Design review of the part built by this model. Coordinates are the model's own, in mm. A direction names the side the tool comes from. Coordinates: 2 decimals unless noted, no trailing zeros. Order: outer loops, then holes, each group sorted by start corner. A loop starts at its lowest first (then second) coordinate and runs counter-clockwise, first axis right, second up. Notation, with made-up numbers: (-15.75, 72.25) -> (23.25, 72.25) arc R17 cw to (23.25, 91.25) -> close; hole circle Ø11 at (-36, 1). An arc over 180 degrees is marked (long way). Use a Markdown table: item, result. Add a question column.
Q1. The part is to be moulded in two halves that separate along X. For faces 4 (the face through (4, 2, 42.9)), 5 (the face through (21.43, 1.68, 23.85)), 6 (the face through (12, 0, 2)), say which applies: pulls with the +X half, pulls with the -X half, needs draft (parallel to the pull), parting line crosses it, or undercut.
Q2. Add section D-D (x = 0.5). Count the separate pieces of the cut face and the enclosed holes in it, then the cut area to 3 significant figures.
Q3. Machinability: for faces 1 (the face through (9.61, 7.53, 23.77)), 2 (the face through (14, -2, 3.5)), 3 (the face through (24, 0, 34.2)), which of the approach directions +Z, -Z, +X, -X, +Y, -Y give a long, thin tool a straight path to every point of the face, cutting with its end or side? Answer none if there is none.
Q4. Insertion check: pin 1 (1.8 mm diameter, centred on x = 13.5, z = 2, fed in from +Y); pin 2 (3 mm diameter, centred on x = 17, z = 17, fed in from +Y); pin 3 (10 mm diameter, centred on x = 14, z = 23, fed in from -Y). Each pin has a flat end and moves straight along its axis. Give the tip position at first contact, or say it passes through.
Q5. Wall thickness on probe 1 along X at (y, z) = (0, 9.25); probe 2 along Z at (x, y) = (8, 6); probe 3 along Y at (x, z) = (22.24, 39.5): over which ranges is each line inside the solid? List them lowest first.
Q6. Add section B-B (x = 16). State the section outline as (y, z) points, then the cut area to 3 significant figures.
Q7. Add section C-C (z = 25.5). State the section outline as (x, y) points, then the cut area to 3 significant figures.
Q8. Add section A-A (z = 7). State the section outline as (x, y) points, then the cut area to 3 significant figures.
from build123d import *

# Parameters (mm, degrees)
SKETCH_1_R          = 1.2
SKETCH_1_R_2        = 0.8
EXTRUDE_3_DEPTH     = 47
SKETCH_6_W          = 5.5
SKETCH_6_H          = 21
CUT_EXTRUDE_4_DEPTH = 53.526968295
SKETCH_7_W          = 15
SKETCH_7_H          = 38.8
CUT_EXTRUDE_5_DEPTH = 56.899041136
CUT_EXTRUDE_6_DEPTH = 56.31273986
CUT_EXTRUDE_7_DEPTH = 56.31273986
SKETCH_10_W         = 38.8
SKETCH_10_H         = 7.6
CUT_EXTRUDE_8_DEPTH = 1
EXTRUDE_4_DEPTH     = 3.5
FILLET_1_R          = 3
SKETCH_12_R         = 3.5
CUT_EXTRUDE_9_DEPTH = 2


with BuildPart() as part:
    # 草图1 → 凸台-拉伸3 (new body)
    with BuildSketch(Plane.XY):
        with BuildLine():
            Line((8.677407083, 12.241756783), (-2.442592917, 2.910968884))
            ThreePointArc((-2.442592917, 2.910968884), (-2.910968884, -2.442592917), (2.442592917, -2.910968884))
            Line((2.442592917, -2.910968884), (11.12, 4.370240199))
            Line((11.12, 4.370240199), (19.797407083, -2.910968884))
            ThreePointArc((19.797407083, -2.910968884), (25.150968884, -2.442592917), (24.682592917, 2.910968884))
            Line((24.682592917, 2.910968884), (13.562592917, 12.241756783))
            ThreePointArc((13.562592917, 12.241756783), (11.12, 13.130787899), (8.677407083, 12.241756783))
        make_face()
        Circle(SKETCH_1_R, mode=Mode.SUBTRACT)
        with Locations((22.24, 0)):
            Circle(SKETCH_1_R_2, mode=Mode.SUBTRACT)
    extrude(amount=EXTRUDE_3_DEPTH)

    # 草图6 → 切除-拉伸4 (cut, through all)
    with BuildSketch(Plane(origin=(11.631625181, 13.862031097, 0), x_dir=(0.7660444431189771, -0.6427876096865404, 0), z_dir=(0.6427876096865404, 0.7660444431189771, 0))):
        with Locations((18.086828415, -23.7)):
            Rectangle(SKETCH_6_W, SKETCH_6_H)
    extrude(amount=-CUT_EXTRUDE_4_DEPTH, mode=Mode.SUBTRACT)

    # 草图7 → 切除-拉伸5 (cut, through all)
    with BuildSketch(Plane(origin=(-2.442592917, 2.910968884, 0), x_dir=(0.766044443118977, 0.6427876096865407, 0), z_dir=(-0.6427876096865407, 0.766044443118977, 0))):
        with Locations((3.7, -23.5)):
            Rectangle(SKETCH_7_W, SKETCH_7_H)
    extrude(amount=-CUT_EXTRUDE_5_DEPTH, mode=Mode.SUBTRACT)

    # 草图8 → 切除-拉伸6 (cut, through all)
    with BuildSketch(Plane.XY.offset(47)):
        with BuildLine():
            Line((19.03136264, -2.268181274), (23.018534178, -3.719393033))
            ThreePointArc((23.018534178, -3.719393033), (21.314980934, -3.685693928), (19.797407083, -2.910968884))
            Line((19.797407083, -2.910968884), (19.03136264, -2.268181274))
        make_face()
    extrude(amount=-CUT_EXTRUDE_6_DEPTH, mode=Mode.SUBTRACT)

    # 草图9 → 切除-拉伸7 (cut, through all)
    with BuildSketch(Plane.XY.offset(47)):
        Polygon((23.018534178, -3.719393033), (12.248842355, 5.317451403), (11.12, 4.370240199), (19.03136264, -2.268181274), align=None)
    extrude(amount=-CUT_EXTRUDE_7_DEPTH, mode=Mode.SUBTRACT)

    # 草图10 → 切除-拉伸8 (cut)
    with BuildSketch(Plane(origin=(8.579697763, 7.199221228, 0), x_dir=(0, 0, 1), z_dir=(-0.7660444431189769, -0.6427876096865407, 0))):
        with Locations((23.5, 0)):
            Rectangle(SKETCH_10_W, SKETCH_10_H)
    extrude(amount=-CUT_EXTRUDE_8_DEPTH, mode=Mode.SUBTRACT)

    # 草图11 → 凸台-拉伸4 (add)
    with BuildSketch(Plane.XY.offset(47)):
        Polygon((0.013310717, -3.799976687), (23.018534178, -3.719393033), (18.585934169, 0), (5.911750542, 0), align=None)
    extrude_4 = extrude(amount=-EXTRUDE_4_DEPTH)

    # 镜向2: 凸台-拉伸4 across plane
    add(extrude_4.mirror(Plane(origin=(0, 0, 23.5), x_dir=(1, 0, 0), z_dir=(0, 0, -1))))

    # 圆角1
    # the kernel refuses this fillet: 3 mm, written as the material it adds along each edge
    with BuildSketch(Plane(origin=(12.248842355, 5.317451403, 47), x_dir=(0.7660444431189768, -0.6427876096865407, 0), z_dir=(0, 0, -1))) as fillet_1_piece_1_section:
        with BuildLine():
            CenterArc((FILLET_1_R * 0.839099631177, FILLET_1_R), FILLET_1_R, 190, 80)
            Line((-FILLET_1_R * 0.145708121835, FILLET_1_R * 0.826351822333), (0, 0))
            Line((0, 0), (FILLET_1_R * 0.839099631177, 0))
        make_face()
    fillet_1_piece_1 = extrude(amount=47, mode=Mode.PRIVATE)
    fillet_1_piece_1 = split(fillet_1_piece_1, bisect_by=Plane(origin=(12.660529152, 4.67576924, 42.9), z_dir=(0, 0, 1)), keep=Keep.TOP, mode=Mode.PRIVATE)
    fillet_1_piece_1 = split(fillet_1_piece_1, bisect_by=Plane(origin=(12.274400975, 4.351769229, 44.95), z_dir=(0.7660444431189769, 0.6427876096865407, 0)), keep=Keep.TOP, mode=Mode.PRIVATE)
    add(fillet_1_piece_1)
    with BuildSketch(Plane(origin=(12.248842355, 5.317451403, 47), x_dir=(0.7660444431189768, -0.6427876096865407, 0), z_dir=(0, 0, -1))) as fillet_1_piece_2_section:
        with BuildLine():
            CenterArc((FILLET_1_R * 0.839099631177, FILLET_1_R), FILLET_1_R, 190, 80)
            Line((-FILLET_1_R * 0.145708121835, FILLET_1_R * 0.826351822333), (0, 0))
            Line((0, 0), (FILLET_1_R * 0.839099631177, 0))
        make_face()
    fillet_1_piece_2 = extrude(amount=47, mode=Mode.PRIVATE)
    fillet_1_piece_2 = split(fillet_1_piece_2, bisect_by=Plane(origin=(11.44751572, 4.445896391, 42.9), z_dir=(0, 0, 1)), keep=Keep.TOP, mode=Mode.PRIVATE)
    fillet_1_piece_2 = split(fillet_1_piece_2, bisect_by=Plane(origin=(11.886403327, 4.81416682, 44.95), z_dir=(-0.7660444431189769, -0.6427876096865407, 0)), keep=Keep.TOP, mode=Mode.PRIVATE)
    add(fillet_1_piece_2)
    with BuildSketch(Plane(origin=(12.248842355, 5.317451403, 47), x_dir=(0.7660444431189768, -0.6427876096865407, 0), z_dir=(0, 0, -1))) as fillet_1_piece_3_section:
        with BuildLine():
            CenterArc((FILLET_1_R * 0.839099631177, FILLET_1_R), FILLET_1_R, 190, 80)
            Line((-FILLET_1_R * 0.145708121835, FILLET_1_R * 0.826351822333), (0, 0))
            Line((0, 0), (FILLET_1_R * 0.839099631177, 0))
        make_face()
    fillet_1_piece_3 = extrude(amount=47, mode=Mode.PRIVATE)
    fillet_1_piece_3 = split(fillet_1_piece_3, bisect_by=Plane(origin=(12.660529152, 4.67576924, 42.9), z_dir=(0, 0, -1)), keep=Keep.TOP, mode=Mode.PRIVATE)
    fillet_1_piece_3 = split(fillet_1_piece_3, bisect_by=Plane(origin=(12.274400975, 4.351769229, 23.5), z_dir=(0.7660444431189769, 0.6427876096865407, 0)), keep=Keep.TOP, mode=Mode.PRIVATE)
    fillet_1_piece_3 = split(fillet_1_piece_3, bisect_by=Plane(origin=(12.660529152, 4.67576924, 4.1), z_dir=(0, 0, 1)), keep=Keep.TOP, mode=Mode.PRIVATE)
    add(fillet_1_piece_3)
    with BuildSketch(Plane(origin=(12.248842355, 5.317451403, 47), x_dir=(0.7660444431189768, -0.6427876096865407, 0), z_dir=(0, 0, -1))) as fillet_1_piece_4_section:
        with BuildLine():
            CenterArc((FILLET_1_R * 0.839099631177, FILLET_1_R), FILLET_1_R, 190, 80)
            Line((-FILLET_1_R * 0.145708121835, FILLET_1_R * 0.826351822333), (0, 0))
            Line((0, 0), (FILLET_1_R * 0.839099631177, 0))
        make_face()
    fillet_1_piece_4 = extrude(amount=47, mode=Mode.PRIVATE)
    fillet_1_piece_4 = split(fillet_1_piece_4, bisect_by=Plane(origin=(12.274400975, 4.351769229, 2.05), z_dir=(0.7660444431189769, 0.6427876096865407, 0)), keep=Keep.TOP, mode=Mode.PRIVATE)
    fillet_1_piece_4 = split(fillet_1_piece_4, bisect_by=Plane(origin=(12.660529152, 4.67576924, 4.1), z_dir=(0, 0, -1)), keep=Keep.TOP, mode=Mode.PRIVATE)
    add(fillet_1_piece_4)
    with BuildSketch(Plane(origin=(12.248842355, 5.317451403, 47), x_dir=(0.7660444431189768, -0.6427876096865407, 0), z_dir=(0, 0, -1))) as fillet_1_piece_5_section:
        with BuildLine():
            CenterArc((FILLET_1_R * 0.839099631177, FILLET_1_R), FILLET_1_R, 190, 80)
            Line((-FILLET_1_R * 0.145708121835, FILLET_1_R * 0.826351822333), (0, 0))
            Line((0, 0), (FILLET_1_R * 0.839099631177, 0))
        make_face()
    fillet_1_piece_5 = extrude(amount=47, mode=Mode.PRIVATE)
    fillet_1_piece_5 = split(fillet_1_piece_5, bisect_by=Plane(origin=(11.886403327, 4.81416682, 2.05), z_dir=(-0.7660444431189769, -0.6427876096865407, 0)), keep=Keep.TOP, mode=Mode.PRIVATE)
    fillet_1_piece_5 = split(fillet_1_piece_5, bisect_by=Plane(origin=(11.44751572, 4.445896391, 4.1), z_dir=(0, 0, -1)), keep=Keep.TOP, mode=Mode.PRIVATE)
    add(fillet_1_piece_5)

    # 草图12 → 切除-拉伸9 (cut)
    with BuildSketch(Plane.XY.offset(4.1)):
        with Locations((5.5, -3.780757684)):
            Circle(SKETCH_12_R)
    extrude(amount=-CUT_EXTRUDE_9_DEPTH, mode=Mode.SUBTRACT)


solid = part.part
Established:
| question | item | result |
|---|---|---|
| 1 | face 4 | needs draft |
| 1 | face 5 | pulls with the +X half |
| 1 | face 6 | undercut |
| 2 | separate pieces | 4 |
| 2 | enclosed holes | 0 |
| 2 | area | 57.3 mm^2 |
| 3 | face 1 | -X, -Y |
| 3 | face 2 | -Y |
| 3 | face 3 | +X, -Y |
| 4 | pin 1 | y = 12.83 |
| 4 | pin 2 | y = 10.62 |
| 4 | pin 3 | y = -0.35 |
| 5 | probe 1 | 18.59 to 21.44, 23.04 to 26.04 |
| 5 | probe 2 | 0 to 4.1, 42.9 to 47 |
| 5 | probe 3 | -3.07 to -0.8, 0.8 to 4.96 |
| 6 | outline | (-3.74, 0) -> (0, 0) -> (0, 3.5) -> (-3.74, 3.5) -> close; (-3.74, 43.5) -> (0, 43.5) -> (0, 47) -> (-3.74, 47) -> close; (2.17, 0) -> (10.2, 0) -> (10.2, 47) -> (2.17, 47) -> close |
| 6 | area | 403 mm^2 |
| 7 | outline | (6.9, 10.75) -> (12.23, 4.4) arc R3 cw to (14.18, 3.7) -> (19.43, -0.71) -> (23.38, 4) -> (13.56, 12.24) arc R3.8 ccw to (8.68, 12.24) -> close |
| 7 | area | 100 mm^2 |
| 8 | outline | (6.9, 10.75) -> (12.23, 4.4) arc R3 cw to (14.18, 3.7) -> (23.02, -3.72) arc R3.8 ccw to (24.68, 2.91) -> (13.56, 12.24) arc R3.8 ccw to (8.68, 12.24) -> close; hole circle Ø1.6 at (22.24, 0) |
| 8 | area | 128 mm^2 |
